Verification items for the finished model (mm, model axes). Give positions to 0.01 mm unless a question says otherwise; leave off trailing zeros. Write each loop counter-clockwise with the first axis right and the second up, starting at its lowest first coordinate (ties: lowest second). Pieces come first, ordered by that corner, then holes. Notation, with made-up numbers: (6.25, 37) -> (30.25, 37) arc R14 cw to (30.25, 56) -> close; hole circle Ø10 at (13, 87). An arc over 180 degrees is marked (long way). Write item = value, one per line.
Autodesk Inventor part; units mm, degrees
ref_plane "YZ Plane" through (0, 0, 0) normal (1, 0, 0) x (0, 1, 0)
ref_plane "XZ Plane" through (0, 0, 0) normal (0, 1, 0) x (-1, 0, 0)
ref_plane "XY Plane" through (0, 0, 0) normal (0, 0, 1) x (1, 0, 0)
sketch "Sketch2" plane through (0, 0, 0) normal (0, 0, 1) x (1, 0, 0)
  circle A0 centre (-57.15, -7.5944) radius 2.3114
  circle A1 centre (-44.45, -7.5944) radius 2.3114
  circle A2 centre (-31.75, -34.1628) radius 2.3114
  circle A3 centre (0.0154, -27.8287) radius 41.275 construction
  line L0 (-52.827, -2.4128) -> (-63.5, -2.4128)
  line L1 (-41.0824, -38.6529) -> (-71.9025, -7.8329)
  circle A4 centre (-63.5, -15.1128) radius 0.7938 construction
  circle A5 centre (-38.1, -40.5128) radius 0.7937 construction
  line L2 (-36.5923, -40.5128) -> (-11.9627, -40.5128)
  line L3 (-69.6574, -2.4128) -> (-45.0278, -2.4128)
  line L4 (-40.5377, -4.2727) -> (-9.7176, -35.0927)
  arc A6 (-69.6574, -2.4128) -> (-71.9025, -7.8329) centre (-69.6574, -5.5878) ccw
  arc A7 (-11.9627, -40.5128) -> (-9.7176, -35.0927) centre (-11.9627, -37.3378) ccw
  arc A8 (-40.5377, -4.2727) -> (-45.0278, -2.4128) centre (-45.0278, -8.7628) ccw
  arc A9 (-41.0824, -38.6529) -> (-36.5923, -40.5128) centre (-36.5923, -34.1628) ccw
  point P0 (-39.2225, -40.5128)
  point P1 (-77.3225, -2.4128)
  point P2 (-4.2975, -40.5128)
  point P3 (-42.3975, -2.4128)
  dimension "d19" = 1.5875
  dimension "d20" = 1.5875
  dimension "d21" = 34.925
  dimension "d22" = 34.925
  dimension "d23" = 3.175
  dimension "d24" = 6.35
  dimension "d25" = 6.35
  dimension "d28" = 82.55
  dimension "d29" = 38.1
  dimension "d30" = 25.4159
  dimension "d31" = 0
  dimension "d32" = 0
  dimension "d33" = 12.0187
  dimension "d34" = 7.3747
  dimension "d35" = 14.9217
extrude "Extrusion2" add sketch "Sketch2" along normal blind 1.5875 contours A1 | L3 A8 L4 A7 L2 A9 L1 A6 L0
sketch "Sketch3" plane through (0, 0, 1.5875) normal (0, 0, 1) x (1, 0, 0)
  line L0 (-71.9025, -7.8329) -> (-41.0824, -38.6529)
  arc A0 (-41.0824, -38.6529) -> (-36.5923, -40.5128) centre (-36.5923, -34.1628) ccw
  line L1 (-36.5923, -40.5128) -> (-11.9627, -40.5128)
  arc A1 (-11.9627, -40.5128) -> (-9.7176, -35.0927) centre (-11.9627, -37.3378) ccw
  line L2 (-9.7176, -35.0927) -> (-40.5377, -4.2727)
  arc A2 (-40.5377, -4.2727) -> (-45.0278, -2.4128) centre (-45.0278, -8.7628) ccw
  line L3 (-45.0278, -2.4128) -> (-69.6574, -2.4128)
  arc A3 (-69.6574, -2.4128) -> (-71.9025, -7.8329) centre (-69.6574, -5.5878) ccw
  circle A4 centre (-31.75, -34.1628) radius 2.3114
  circle A5 centre (-57.15, -7.5944) radius 2.3114
  point P0 (0, 0)
equation "\"BendRadius\" = Thickness"
equation "\"BendReliefWidth\" = Thickness"
equation "\"BendReliefDepth\" = 0.5 * Thickness"
equation "\"CornerReliefSize\" = 4 * Thickness"
equation "\"MinimumRemnant\" = 2 * Thickness"
equation "\"TransitionRadius\" = BendRadius"
equation "\"JacobiRadiusSize\" = BendRadius"
equation "\"GapSize\" = Thickness"
properties part number "chrissled" material "Polycarbonate, Clear"
Item 1: Mould release check, pull along X, two halves, no side actions. Record for faces 1 (the flat face through (-41, -21, 0)), 2 (the cylindrical face through (-72.6, -4.4, 0.8)), 3 (the cylindrical face through (-58.984, -6.188, 0.783)): +X half, -X half, draft (parallel to the pull), parting line (faces both ways), or undercut.
Response values:
face_1 = draft
face_2 = -X half
face_3 = undercut
Item 2: Sectioned sample at D-D on y = -26. Record the cut outline in (x, z).
Response values:
outline = (-53.74, 0) -> (-18.81, 0) -> (-18.81, 1.59) -> (-53.74, 1.59) -> close
Item 3: Sectioned sample at B-B on x = -31.75. Record the cut outline in (y, z).
Response values:
outline = (-40.51, 0) -> (-36.47, 0) -> (-36.47, 1.59) -> (-40.51, 1.59) -> close; (-31.85, 0) -> (-13.06, 0) -> (-13.06, 1.59) -> (-31.85, 1.59) -> close
Item 4: Material ranges on line 1 (Y direction, x = -31.75, z = 1.2); line 2 (Y direction, x = -33.5, z = 0.9); line 3 (X direction, y = -7, z = 0.95), recorded low to high.
Response values:
line_1 = -40.51 to -36.47, -31.85 to -13.06
line_2 = -40.51 to -35.67, -32.65 to -11.31
line_3 = -72.5 to -59.38, -54.92 to -37.81
Item 5: Sectioned sample at C-C on x = -66.5. Record the cut outline in (y, z), then the cut area to 3 significant figures.
Response values:
outline = (-13.24, 0) -> (-2.41, 0) -> (-2.41, 1.59) -> (-13.24, 1.59) -> close
area = 17.2 mm^2
Item 6: Sectioned sample at A-A on x = -57.15. Record the cut outline in (y, z), then the cut area to 3 significant figures.
Response values:
outline = (-22.59, 0) -> (-9.91, 0) -> (-9.91, 1.59) -> (-22.59, 1.59) -> close; (-5.28, 0) -> (-2.41, 0) -> (-2.41, 1.59) -> (-5.28, 1.59) -> close
area = 24.7 mm^2
